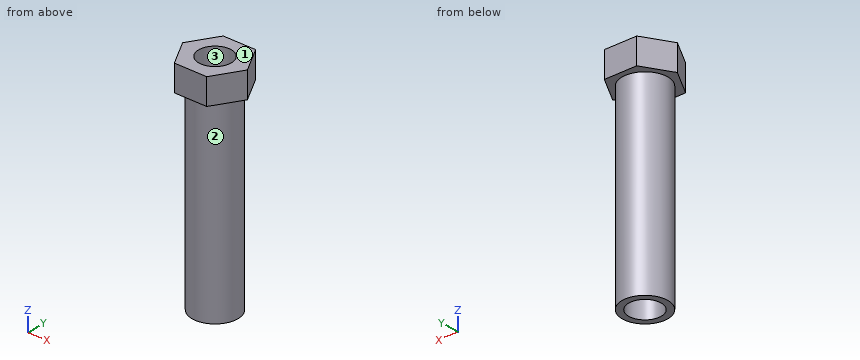
```python
from build123d import *

# Parameters (mm, degrees)
EXTRUDE_1_DEPTH     = 4
SKETCH_2_R          = 3.5
SKETCH_2_R_2        = 2.5
EXTRUDE_2_DEPTH     = 30
SKETCH_3_R          = 2.5
CUT_EXTRUDE_1_DEPTH = 64


with BuildPart() as part:
    # 草图1 → 凸台-拉伸1 (new body)
    with BuildSketch(Plane.XY):
        Polygon((5.051814855, 0), (2.525907428, 4.375), (-2.525907428, 4.375), (-5.051814855, 0), (-2.525907428, -4.375), (2.525907428, -4.375), align=None)
    extrude(amount=EXTRUDE_1_DEPTH)

    # 草图2 → 凸台-拉伸2 (add)
    with BuildSketch(Plane(origin=(0, 0, 0), x_dir=(-1, 0, 0), z_dir=(0, 0, -1))):
        Circle(SKETCH_2_R)
        Circle(SKETCH_2_R_2, mode=Mode.SUBTRACT)
    extrude(amount=EXTRUDE_2_DEPTH)

    # 草图3 → 切除-拉伸1 (cut)
    with BuildSketch(Plane.XY.offset(4)):
        Circle(SKETCH_3_R)
    extrude(amount=-CUT_EXTRUDE_1_DEPTH, mode=Mode.SUBTRACT)


solid = part.part
```
Input: part model. Units: mm. Frame: model coordinates. Face numbers are marked on the shaded views. Coordinates: 2 decimals unless noted, no trailing zeros. Order: outer loops, then holes, each group sorted by start corner. A loop starts at its lowest first (then second) coordinate and runs counter-clockwise, first axis right, second up. Notation, with made-up numbers: (40.25, -10) - (85.25, -10) arc R21 cw to (85.25, 3) - close; hole circle Ø1 at (28, -15). An arc over 180 degrees is marked (long way). Return JSON: item names as keys, results as strings.
Q1. Cut plane D-D (x = 3). Return loops of the section in (y, z).
The answers:
{"outline": "(-3.55, 0) - (-1.8, 0) - (-1.8, -30) - (1.8, -30) - (1.8, 0) - (3.55, 0) - (3.55, 4) - (-3.55, 4) - close"}
Q2. Cut plane A-A (x = 0). Return loops of the section in (y, z) (3 decimals).
The answers:
{"outline": "(-4.375, 0) - (-3.5, 0) - (-3.5, -30) - (-2.5, -30) - (-2.5, 4) - (-4.375, 4) - close; (2.5, -30) - (3.5, -30) - (3.5, 0) - (4.375, 0) - (4.375, 4) - (2.5, 4) - close"}
Q3. Cut plane B-B (y = 2). Return loops of the section in (x, z), then the cut area to 3 significant figures.
The answers:
{"outline": "(-3.9, 0) - (-2.87, 0) - (-2.87, -30) - (-1.5, -30) - (-1.5, 4) - (-3.9, 4) - close; (1.5, -30) - (2.87, -30) - (2.87, 0) - (3.9, 0) - (3.9, 4) - (1.5, 4) - close", "area": "102 mm2"}
Q4. Cut plane C-C (z = -21.5). Return loops of the section in (x, y).
The answers:
{"outline": "circle Ø7 at (0, 0); hole circle Ø5 at (0, 0)"}
Q5. First-contact query: pin 1 (6 mm diameter, centred on x = -2, z = -18.5, fed in from +Y); pin 2 (3 mm diameter, centred on y = 1, z = -0.5, fed in from +X); pin 3 (1.5 mm diameter, centred on x = -1.5, y = 0.5, fed in from -Z); pin 4 (3 mm diameter, centred on x = 3.5, z = -22, fed in from +Y). Flat tips, straight axial feed; report the tip coordinate or a pass-through.
The answers:
{"pin 1": "stops at y = 3.5", "pin 2": "stops at x = 5.05", "pin 3": "passes through", "pin 4": "stops at y = 2.87"}
Q6. Draft query along X for the marked faces 1, 2 and 3. Return one class per face: +X half, -X half, draft (parallel to the pull), parting line (faces both ways), or undercut.
The answers:
{"face 1": "draft", "face 2": "parting line", "face 3": "undercut"}
Q7. Ray query, probe 1 along Y at (x, z) = (0, -15.5); probe 2 along Z at (x, y) = (-3, -2.5); probe 3 along X at (y, z) = (0.75, 1). Return the intervals inside material, ascending.
The answers:
{"probe 1": "y = -3.5 to -2.5, 2.5 to 3.5", "probe 2": "z = 0 to 4", "probe 3": "x = -4.62 to -2.38, 2.38 to 4.62"}
